from build123d import *

# Parameters (mm, degrees)
F0_W     = 20
F0_H     = 20
F0_R     = 8
F0_R_2   = 7
F0_R_3   = 0.75
F1_DEPTH = 10
F2_R     = 1.25
F3_DEPTH = 25
F4_DEPTH = 6
F5_R     = 1.25
F5_R_2   = 0.75
F6_DEPTH = 5


with BuildPart() as f1:
    # F0 (on Top) → F1 (new body)
    with BuildSketch(Plane.XY):
        with Locations((10, -10)):
            Rectangle(F0_W, F0_H)
        with Locations((10, -10)):
            Circle(F0_R, mode=Mode.SUBTRACT)
        with Locations((10, -10)):
            Circle(F0_R)
        with Locations((10, -10)):
            Circle(F0_R_2, mode=Mode.SUBTRACT)
        with Locations((10, -10)):
            Circle(F0_R_2)
        with Locations((10, -14.25)):
            Circle(F0_R_3, mode=Mode.SUBTRACT)
        with Locations((5.75, -10)):
            Circle(F0_R_3, mode=Mode.SUBTRACT)
        with Locations((14.25, -10)):
            Circle(F0_R_3, mode=Mode.SUBTRACT)
        with Locations((10, -5.75)):
            Circle(F0_R_3, mode=Mode.SUBTRACT)
        with Locations((10, -14.25)):
            Circle(F0_R_3)
        with Locations((10, -5.75)):
            Circle(F0_R_3)
    extrude(amount=-F1_DEPTH)

    # F2 (on face) → F3 (cut)
    with BuildSketch(Plane(origin=(0, 0, 0), x_dir=(0, -1, 0), z_dir=(-1, 0, 0))):
        with Locations((5.75, -5)):
            Circle(F2_R)
        with Locations((14.25, -5)):
            Circle(F2_R)
    extrude(amount=-F3_DEPTH, mode=Mode.SUBTRACT)

    # F0 (on Top) → F4 (cut)
    with BuildSketch(Plane.XY):
        with Locations((10, -5.75)):
            Circle(F0_R_3)
        with Locations((10, -14.25)):
            Circle(F0_R_3)
    extrude(amount=-F4_DEPTH, mode=Mode.SUBTRACT)

    # F5 (on face) → F6 (cut)
    with BuildSketch(Plane(origin=(0, 0, -10), x_dir=(1, 0, 0), z_dir=(0, 0, -1))):
        with Locations((5.75, 10)):
            Circle(F5_R)
        with Locations((5.75, 10)):
            Circle(F5_R_2, mode=Mode.SUBTRACT)
        with Locations((14.25, 10)):
            Circle(F5_R)
        with Locations((14.25, 10)):
            Circle(F5_R_2, mode=Mode.SUBTRACT)
    extrude(amount=-F6_DEPTH, mode=Mode.SUBTRACT)


solid = f1.part
CAD build for the part. Positions are in the model's coordinates, mm. A direction names the side the tool comes from. Round coordinates to 2 decimals unless told otherwise and drop trailing zeros. Order: outer loops, then holes, each group sorted by start corner. A loop starts at its lowest first (then second) coordinate and runs counter-clockwise, first axis right, second up. Notation, with made-up numbers: M 27,45.5 L 61,45.5 A16 cw 61,75.5 Z; hole C 71,77 d9. An arc over 180 degrees is marked long. Use one line per item in the form item = value.
Q1. Saw through at A-A on x = 5.75. Give the cut face in (y, z).
Recorded:
outline = M -20,-10 L -11.25,-10 L -11.25,-5 L -10.75,-5 L -10.75,0 L -20,0 Z; M -9.25,-5 L -8.75,-5 L -8.75,-10 L 0,-10 L 0,0 L -9.25,0 Z; hole C -14.25,-5 d2.5; hole C -5.75,-5 d2.5
Q2. Probe L1, parallel to X at y = -10, z = -6.8; L2, parallel to Y at x = 16, z = -4; L3, parallel to X at y = -9.5, z = -7. List the from-to ranges inside material, lowest first.
Recorded:
L1 = 0 to 4.5, 7 to 13, 15.5 to 20
L2 = -20 to -15, -13.5 to -6.5, -5 to 0
L3 = 0 to 4.6, 6.9 to 13.1, 15.4 to 20
Q3. Saw through at C-C on z = -1.25. Give the cut face in (x, y), then the cut area to 3 significant figures.
Recorded:
outline = M 0,-20 L 20,-20 L 20,0 L 0,0 Z; hole C 5.75,-10 d1.5; hole C 10,-14.25 d1.5; hole C 10,-5.75 d1.5; hole C 14.25,-10 d1.5
area = 393 mm^2
Q4. Saw through at D-D on x = 2.25. Give the cut face in (y, z).
Recorded:
outline = M -20,-10 L 0,-10 L 0,0 L -20,0 Z; hole C -14.25,-5 d2.5; hole C -5.75,-5 d2.5
Q5. Which spindle directions (+Z, -Z, +X, -X, +Y, -Y) get a long thin tool onto all of the face, cutting with end or side? Do faces 1 (the cylindrical face through (14.09, -11.24, -7.54)), 2 (the cylindrical face through (13.7, -9.49, -2.46)), 3 (the cylindrical face through (9.45, -13.74, -1.97)). Say none if no direction does.
Recorded:
face_1 = -Z
face_2 = +Z, -Z
face_3 = +Z
Q6. Two-plate mould, pull along X, no slides. Class faces 4 (the flat face through (10, 0, -5)), 5 (the flat face through (6, -9, -5)), 6 (the flat face through (0, -10, -5)): +X half, -X half, draft (parallel to the pull), parting line (faces both ways), or undercut.
Recorded:
face_4 = draft
face_5 = undercut
face_6 = -X half
Q7. Flat gauge pins, fed straight in: P1, Ø3, axis at x = 5.75, y = -10, coming from the -Z side; P2, Ø1.2, axis at x = 14, y = -10.5, coming from the -Z side; P3, Ø1.4, axis at x = 10, y = -14.25, coming from the +Z side. Where does each tip first touch, or does it go through?
Recorded:
P1 = -10
P2 = -5
P3 = -6.04
Q8. Saw through at B-B on y = -5.75. Give the cut face in (x, z), then the cut area to 3 significant figures.
Recorded:
outline = M 0,-10 L 20,-10 L 20,-6.25 L 0,-6.25 Z; M 0,-3.75 L 9.25,-3.75 L 9.25,0 L 0,0 Z; M 10.75,-3.75 L 20,-3.75 L 20,0 L 10.75,0 Z
area = 144 mm^2
